Autodesk Inventor part; units mm, degrees
ref_plane "YZ Plane" through (0, 0, 0) normal (1, 0, 0) x (0, 1, 0)
ref_plane "XZ Plane" through (0, 0, 0) normal (0, 1, 0) x (-1, 0, 0)
ref_plane "XY Plane" through (0, 0, 0) normal (0, 0, 1) x (1, 0, 0)
sketch "スケッチ1" plane through (0, 0, 0) normal (1, 0, 0) x (0, 1, 0)
  circle A0 centre (0, 0) radius 20
  dimension "d0" = 40
extrude "押し出し1" add sketch "スケッチ1" along normal blind 53.6
sketch "スケッチ2" plane through (53.6, 0, 0) normal (1, 0, 0) x (0, 0, -1)
  circle A0 centre (0, 0) radius 22
  dimension "d3" = 44
extrude "押し出し2" add sketch "スケッチ2" along normal blind 1
sketch "スケッチ3" plane through (54.6, 0, 0) normal (1, 0, 0) x (0, 0, -1)
  circle A0 centre (0, 0) radius 7
  dimension "d6" = 14
extrude "押し出し3" add sketch "スケッチ3" along normal blind 1
sketch "スケッチ4" plane through (0, 0, 0) normal (-1, 0, 0) x (0, 0, 1)
  circle A0 centre (0, 0) radius 22
  dimension "d9" = 44
extrude "押し出し4" add sketch "スケッチ4" along normal blind 1
sketch "スケッチ5" plane through (-1, 0, 0) normal (-1, 0, 0) x (0, 0, 1)
  circle A0 centre (0, 0) radius 7
  dimension "d12" = 14
extrude "押し出し5" add sketch "スケッチ5" along normal blind 1
sketch "スケッチ6" plane through (55.6, 0, 0) normal (1, 0, 0) x (0, 0, -1)
  circle A0 centre (0, 0) radius 7
hole "穴1" at (55.6, 0, 0) direction (-1, 0, 0) diameter 10.2 end through all
properties part number "CLS_typeC_31.4N"
Source: CAD feature listing. Evaluate the final solid. Frame: model axes, mm. A direction names the side the tool comes from. Round coordinates to 2 decimals unless told otherwise and drop trailing zeros. Loops run counter-clockwise (first coordinate to the right, second up) from the corner with the lowest first, then second, coordinate; pieces in that order, holes last. Notation, with made-up numbers: (79, 36) - (130, 36) arc R37 ccw to (130, 74) - close; hole circle Ø1 at (-27.75, 5). An arc over 180 degrees is marked (long way). Write item = value, one per line. Start each with the question number.
Item 1: Section query D-D on y = -14. Output: boundary loops of the cut face in (x, z).
Item 2: Material intervals for line 1 (Z direction, x = 13, y = 0); line 2 (X direction, y = 9, z = 19); line 3 (X direction, y = 2.5, z = -15), sorted ascending.
Item 3: Section query C-C on x = 12.5. Output: boundary loops of the cut face in (y, z).
Item 4: Section query A-A on y = 0. Output: boundary loops of the cut face in (x, z).
Item 5: First-contact query: pin 1 Ø4 at (x, y) = (47.5, 1) entering from -Z; pin 2 Ø5 at (x, z) = (28.5, -3) entering from -Y; pin 3 Ø5 at (x, z) = (27, -5) entering from +Y. Flat tips, straight axial feed; report the tip coordinate or a pass-through.
Item 6: Mould query, pull axis X, two halves, no side actions, for faces 6 (the face through (26.425, -4.336, 19.524)), 7 (the face through (54.6, 5.2, 5.2)), 8 (the face through (-1, 5.2, -5.2)). Classes: released by +X, released by -X, zero draft, split by the parting line, or undercut.
Item 7: Reachability of faces 1 (the face through (0, -18, 10)), 2 (the face through (-1.493, 2.681, 6.466)), 3 (the face through (-2, -2, -5)), 4 (the face through (54.093, 21.477, 4.769)), 5 (the face through (55.093, 2.681, -6.466)) from +Z, -Z, +X, -X, +Y, -Y: full face, straight path, thin tool, end or side. Return the list, or none.
Results list:
q1.outline = (-1, -16.97) - (0, -16.97) - (0, -14.28) - (53.6, -14.28) - (53.6, -16.97) - (54.6, -16.97) - (54.6, 16.97) - (53.6, 16.97) - (53.6, 14.28) - (0, 14.28) - (0, 16.97) - (-1, 16.97) - close
q2.line_1 = -20 to -5.1, 5.1 to 20
q2.line_2 = -1 to 0, 53.6 to 54.6
q2.line_3 = -1 to 54.6
q3.outline = circle Ø40 at (0, 0); hole circle Ø10.2 at (0, 0)
q4.outline = (-2, -7) - (-1, -7) - (-1, -22) - (0, -22) - (0, -20) - (53.6, -20) - (53.6, -22) - (54.6, -22) - (54.6, -7) - (55.6, -7) - (55.6, -5.1) - (-2, -5.1) - close; (-2, 5.1) - (55.6, 5.1) - (55.6, 7) - (54.6, 7) - (54.6, 22) - (53.6, 22) - (53.6, 20) - (0, 20) - (0, 22) - (-1, 22) - (-1, 7) - (-2, 7) - close
q5.pin_1 = -20
q5.pin_2 = -19.99
q5.pin_3 = 19.84
q6.face_6 = undercut
q6.face_7 = released by +X
q6.face_8 = released by -X
q7.face_1 = none
q7.face_2 = -X
q7.face_3 = +Z, -Z, -X, +Y, -Y
q7.face_4 = +X, -X
q7.face_5 = +X
